Here's the drawing with two shaded views (mm, measured from the low corner). I have some questions. Give positions to 0.01 mm unless a question says otherwise; leave off trailing zeros. Write each loop counter-clockwise with the first axis right and the second up, starting at its lowest first coordinate (ties: lowest second). Pieces come first, ordered by that corner, then holes. Notation, with made-up numbers: M 73,-32.5 L 105,-32.5 A20 ccw 105,-11.5 Z; hole C -21.75,78.5 d7. An arc over 180 degrees is marked long. Answer as a JSON object with one key per item and string values. Group by question number.
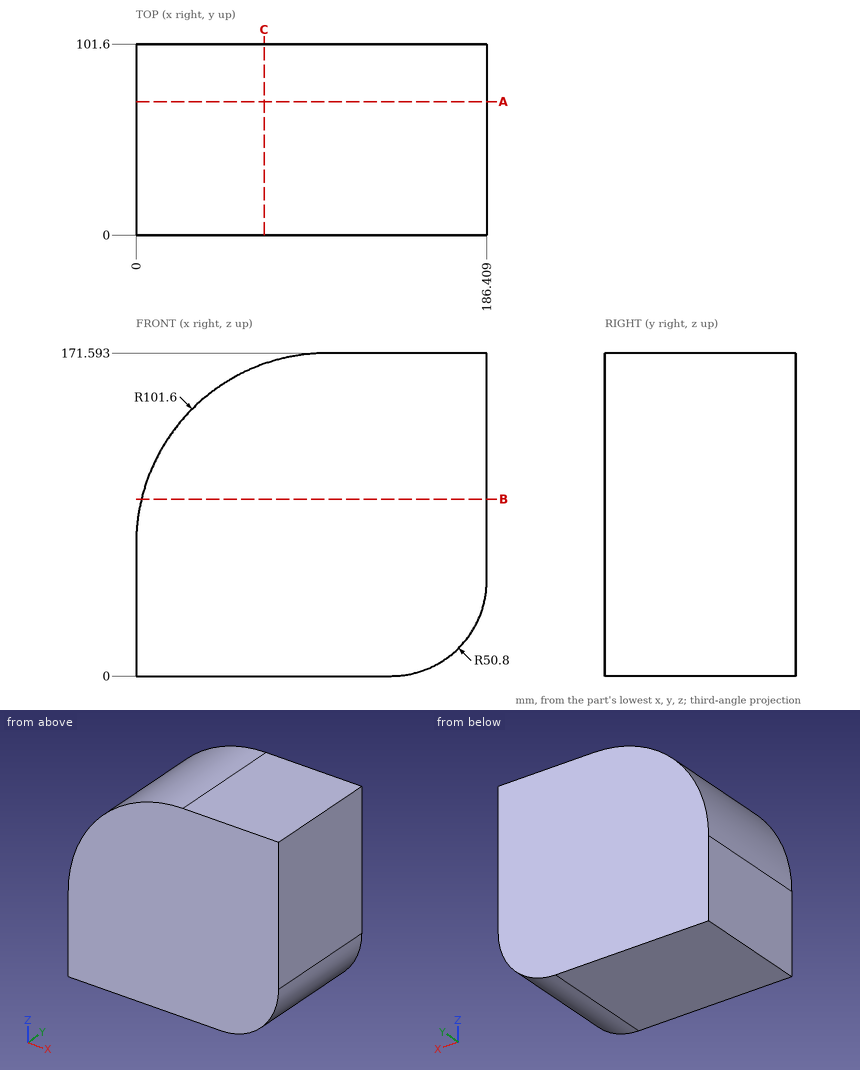
1) Please list where these lines run through material, in increasing order: line 1 along X through (y, z) = (65.5, 49); line 2 along Z through (x, y) = (145, 31) (1 decimal); line 3 along X through (y, z) = (55, 97) (1 decimal). Write a range as from..to.
2) If we section it at A-A, the plane y = 71: List the corners of the cut face in (x, z) for me, plus the area to 3 significant figures.
3) If we section it at B-B, the plane z = 94: List the corners of the cut face in (x, y) for me.
4) If we section it at C-C, the plane x = 68: List the corners of the cut face in (y, z) for me.
5) I'm going to push flat-ended pins straight in: pin 1 (4 mm diameter, centred on x = 22, y = 37, fed in from -Z); pin 2 (2 mm diameter, centred on x = 161.5, y = 14.5, fed in from -Z); pin 3 (10 mm diameter, centred on y = 69.5, z = 149.5, fed in from -X) (1 decimal). Where does each tip first touch, or does it pass through?
Taken from the geometry:
{
 "1": {"line 1": "0..186.38", "line 2": "0.9..171.6", "line 3": "3.7..186.4"},
 "2": {"outline": "M 0,0 L 135.61,0 A50.8 ccw 186.41,50.8 L 186.41,171.59 L 101.6,171.59 A101.6 ccw 0,69.99 Z", "area": "29,200 mm²"},
 "3": {"outline": "M 2.88,0 L 186.41,0 L 186.41,101.6 L 2.88,101.6 Z"},
 "4": {"outline": "M 0,0 L 101.6,0 L 101.6,165.88 L 0,165.88 Z"},
 "5": {"pin 1": "z = 0", "pin 2": "z = 6.52", "pin 3": "x = 32.5"}
}
